Print and shaded views of the part. All mm, measured from the part's lowest x, y and z. A direction names the side the tool comes from. Round coordinates to 2 decimals unless told otherwise and drop trailing zeros. Loops run counter-clockwise (first coordinate to the right, second up) from the corner with the lowest first, then second, coordinate; pieces in that order, holes last. Notation, with made-up numbers: (14.5, -4.5) - (68.5, -4.5) arc R29 cw to (68.5, 31.5) - close; hole circle Ø8 at (49.25, 22.5). An arc over 180 degrees is marked (long way). Use one line per item in the form item = value.
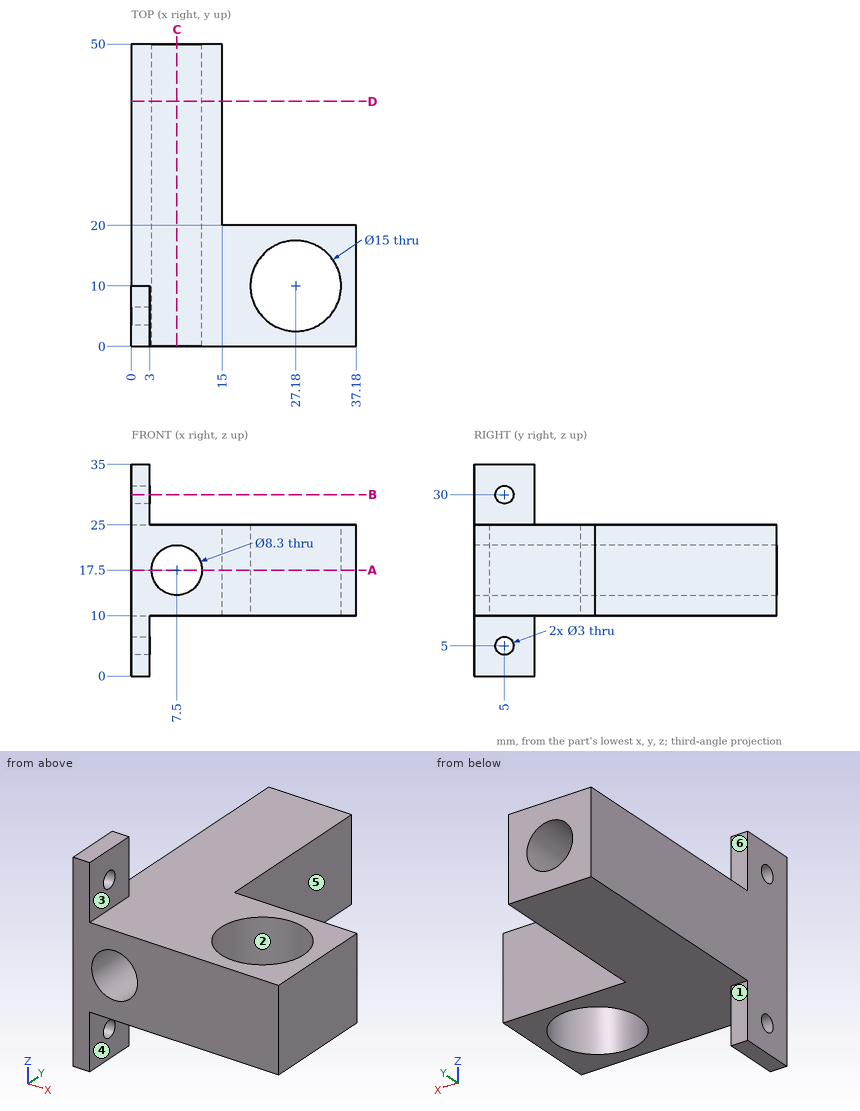
1. Cut at D-D, the plane y = 40.5. Give the cut face in (x, z).
Geometry check:
outline = (0, 10) - (15, 10) - (15, 25) - (0, 25) - close; hole circle Ø8.3 at (7.5, 17.5)
2. Flat gauge pins, fed straight in: pin 1 (4.5 mm diameter, centred on y = 33, z = 18, fed in from +X); pin 2 (18.5 mm diameter, centred on x = 10.5, y = 15.5, fed in from +Z); pin 3 (12 mm diameter, centred on x = 30, y = 14.5, fed in from -Z); pin 4 (13.5 mm diameter, centred on x = 7.5, z = 17.5, fed in from +Y). Where does each tip first touch, or does it go through?
Geometry check:
pin_1 = 15
pin_2 = 25
pin_3 = 10
pin_4 = 50
3. Cut at C-C, the plane x = 7.5. Give the cut face in (y, z).
Geometry check:
outline = (0, 10) - (50, 10) - (50, 13.35) - (0, 13.35) - close; (0, 21.65) - (50, 21.65) - (50, 25) - (0, 25) - close
4. Cut at A-A, the plane z = 17.5. Give the cut face in (x, y), plus the area to 3 significant figures.
Geometry check:
outline = (0, 0) - (3.35, 0) - (3.35, 50) - (0, 50) - close; (11.65, 0) - (37.18, 0) - (37.18, 20) - (15, 20) - (15, 50) - (11.65, 50) - close; hole circle Ø15 at (27.18, 10)
area = 602 mm^2
5. Wall check: probe 1 along X at (y, z) = (37, 11); probe 2 along Y at (x, z) = (35, 14); probe 3 along Z at (x, y) = (6.5, 32). Give the ranges that are in metal, low to high.
Geometry check:
probe_1 = 0 to 15
probe_2 = 0 to 20
probe_3 = 10 to 13.47, 21.53 to 25
6. Cut at B-B, the plane z = 30. Give the cut face in (x, y), plus the area to 3 significant figures.
Geometry check:
outline = (0, 0) - (3, 0) - (3, 3.5) - (0, 3.5) - close; (0, 6.5) - (3, 6.5) - (3, 10) - (0, 10) - close
area = 21.0 mm^2
7. Tool access for the marked faces 4, 5 and 6: list every direction of +Z, -Z, +X, -X, +Y, -Y with a clear straight run to the whole face (end or side of a thin tool).
Geometry check:
face_4 = -Z, +X, +Y, -Y
face_5 = +Z, -Z, +X, +Y
face_6 = +Z, +X, -X, +Y
8. Pull direction X, two halves, no side cores. Call the marked faces 1, 2 and 3: +X half, -X half, draft (parallel to the pull), parting line (faces both ways), or undercut.
Geometry check:
face_1 = draft
face_2 = undercut
face_3 = +X half
